from build123d import *

# Parameters (mm, degrees)
BOSS_EXTRUDE1_DEPTH = 76.2
SKETCH2_R           = 6.86
CUT_EXTRUDE1_DEPTH  = 14.224
SKETCH3_R           = 6.86
CUT_EXTRUDE2_DEPTH  = 14.224
SKETCH4_R           = 3.5
CUT_EXTRUDE3_DEPTH  = 77.2


with BuildPart() as part:
    # Sketch1 → Boss-Extrude1 (new body)
    with BuildSketch(Plane(origin=(0, 0, 0), x_dir=(0, 1, 0), z_dir=(0, 0, 1))):
        Polygon((7.112, -4.106115114), (7.112, 4.106115114), (0, 8.212230229), (-7.112, 4.106115114), (-7.112, -4.106115114), (0, -8.212230229), align=None)
    extrude(amount=BOSS_EXTRUDE1_DEPTH)

    # Sketch2 → Cut-Extrude1 (cut)
    with BuildSketch(Plane.XY.offset(76.2)):
        Polygon((8.212230229, 0), (4.106115114, 7.112), (-4.106115114, 7.112), (-8.212230229, 0), (-4.106115114, -7.112), (4.106115114, -7.112), align=None)
        Circle(SKETCH2_R, mode=Mode.SUBTRACT)
    extrude(amount=-CUT_EXTRUDE1_DEPTH, mode=Mode.SUBTRACT)

    # Sketch3 → Cut-Extrude2 (cut)
    with BuildSketch(Plane(origin=(0, 0, 0), x_dir=(1, 0, 0), z_dir=(0, 0, -1))):
        Polygon((4.106115114, -7.112), (8.212230229, 0), (4.106115114, 7.112), (-4.106115114, 7.112), (-8.212230229, 0), (-4.106115114, -7.112), align=None)
        Circle(SKETCH3_R, mode=Mode.SUBTRACT)
    extrude(amount=-CUT_EXTRUDE2_DEPTH, mode=Mode.SUBTRACT)

    # Sketch4 → Cut-Extrude3 (cut, through all)
    with BuildSketch(Plane(origin=(0, 0, 0), x_dir=(1, 0, 0), z_dir=(0, 0, -1))):
        Circle(SKETCH4_R)
    extrude(amount=-CUT_EXTRUDE3_DEPTH, mode=Mode.SUBTRACT)


solid = part.part
CAD build for the part. Positions are in the model's coordinates, mm. A direction names the side the tool comes from. Give positions to 0.01 mm unless a question says otherwise; leave off trailing zeros. Write each loop counter-clockwise with the first axis right and the second up, starting at its lowest first coordinate (ties: lowest second). Pieces come first, ordered by that corner, then holes. Notation, with made-up numbers: (9, -27) -> (13, -27) arc R24 cw to (13, 1) -> close; hole circle Ø10 at (-4, 4.5). An arc over 180 degrees is marked (long way). Return JSON: item names as keys, results as strings.
Item 1: Drop flat-ended pins along their axis: pin 1 (4 mm diameter, centred on x = 0, y = 0, fed in from +Z); pin 2 (1 mm diameter, centred on x = -1.5, z = 9.5, fed in from +Y); pin 3 (2 mm diameter, centred on y = -3.5, z = 67, fed in from +X); pin 4 (8 mm diameter, centred on y = -3.5, z = 21, fed in from +X). Give the stop position or say it passes through.
Answer below:
{"pin 1": "passes through", "pin 2": "stops at y = 6.79", "pin 3": "stops at x = 6.39", "pin 4": "stops at x = 8.21"}
Item 2: Band-saw the part on A-A (x = 0). List the corners of the cut face in (y, z), then the cut area to 3 significant figures.
Answer below:
{"outline": "(-7.11, 14.22) -> (-6.86, 14.22) -> (-6.86, 0) -> (-3.5, 0) -> (-3.5, 76.2) -> (-6.86, 76.2) -> (-6.86, 61.98) -> (-7.11, 61.98) -> close; (3.5, 0) -> (6.86, 0) -> (6.86, 14.22) -> (7.11, 14.22) -> (7.11, 61.98) -> (6.86, 61.98) -> (6.86, 76.2) -> (3.5, 76.2) -> close", "area": "536 mm2"}
Item 3: Drill centre lines: probe 1 along Y at (x, z) = (0, 49); probe 2 along X at (y, z) = (0, 27.5); probe 3 along Y at (x, z) = (1, 53.5). Where is each one in solid material? Low to high.
Answer below:
{"probe 1": "y = -7.11 to -3.5, 3.5 to 7.11", "probe 2": "x = -8.21 to -3.5, 3.5 to 8.21", "probe 3": "y = -7.11 to -3.35, 3.35 to 7.11"}
Item 4: Tool access for faces 5 (the flat face through (0, 7.112, 38)), 6 (the cylindrical face through (6.543, 2.061, 69.188)), 7 (the flat face through (6.7, -2.1, 14.224)): list every direction of +Z, -Z, +X, -X, +Y, -Y with a clear straight run to the whole face (end or side of a thin tool).
Answer below:
{"face 5": "+Z, -Z, +X, -X, +Y", "face 6": "+Z", "face 7": "-Z"}
Item 5: Band-saw the part on D-D (x = 5). List the corners of the cut face in (y, z).
Answer below:
{"outline": "(-5.56, 14.22) -> (-4.7, 14.22) -> (-4.7, 0) -> (4.7, 0) -> (4.7, 14.22) -> (5.56, 14.22) -> (5.56, 61.98) -> (4.7, 61.98) -> (4.7, 76.2) -> (-4.7, 76.2) -> (-4.7, 61.98) -> (-5.56, 61.98) -> close"}
Item 6: Band-saw the part on C-C (y = -1.5). List the corners of the cut face in (x, z), then the cut area to 3 significant figures.
Answer below:
{"outline": "(-7.35, 14.22) -> (-6.69, 14.22) -> (-6.69, 0) -> (-3.16, 0) -> (-3.16, 76.2) -> (-6.69, 76.2) -> (-6.69, 61.98) -> (-7.35, 61.98) -> close; (3.16, 0) -> (6.69, 0) -> (6.69, 14.22) -> (7.35, 14.22) -> (7.35, 61.98) -> (6.69, 61.98) -> (6.69, 76.2) -> (3.16, 76.2) -> close", "area": "601 mm2"}
Item 7: Two-plate mould, pull along X, no slides. Class faces 1 (the cylindrical face through (6.543, -2.061, 7.012)), 2 (the cylindrical face through (3.233, 1.341, 37.567)), 3 (the flat face through (-6.188, -3.506, 37.766)), 4 (the flat face through (3, 3, 0)): +X half, -X half, draft (parallel to the pull), parting line (faces both ways), or undercut.
Answer below:
{"face 1": "parting line", "face 2": "undercut", "face 3": "-X half", "face 4": "draft"}
Item 8: Band-saw the part on B-B (z = 57). List the corners of the cut face in (x, y), then the cut area to 3 significant figures.
Answer below:
{"outline": "(-8.21, 0) -> (-4.11, -7.11) -> (4.11, -7.11) -> (8.21, 0) -> (4.11, 7.11) -> (-4.11, 7.11) -> close; hole circle Ø7 at (0, 0)", "area": "137 mm2"}
